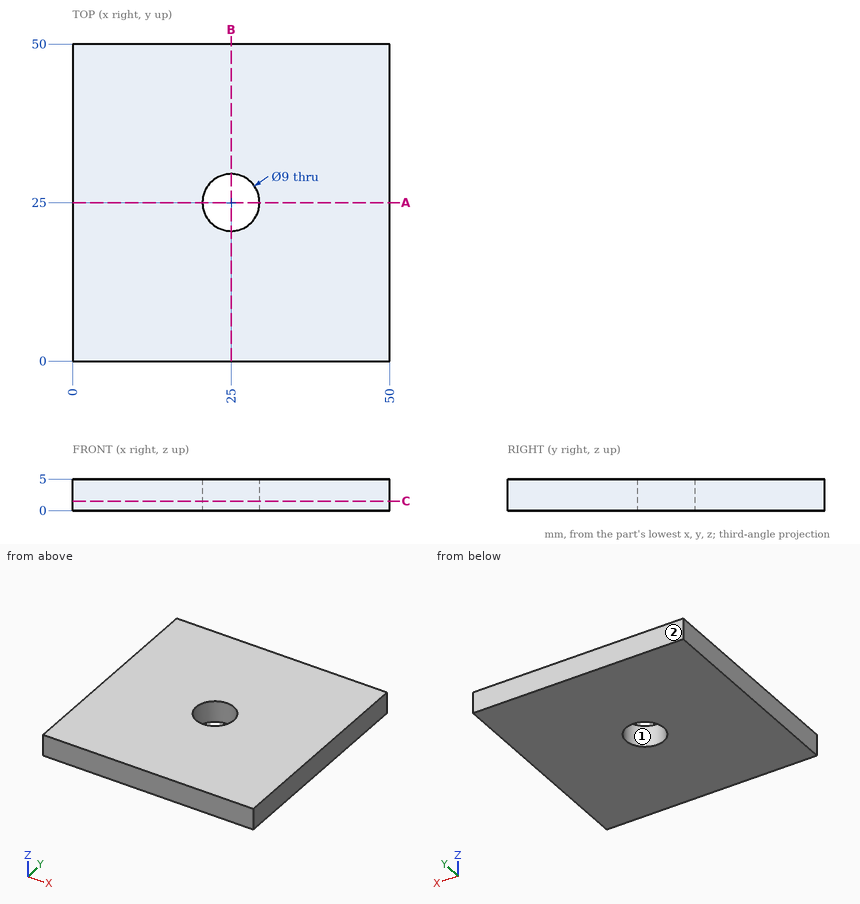
Drawing for the job (mm, zero at the part's lowest x, y, z). Give positions to 0.01 mm unless a question says otherwise; leave off trailing zeros. Loops run counter-clockwise (first coordinate to the right, second up) from the corner with the lowest first, then second, coordinate; pieces in that order, holes last. Notation, with made-up numbers: (-13, 76.5) - (18, 76.5) arc R14 cw to (18, 94.5) - close; hole circle Ø3 at (31, -25). An arc over 180 degrees is marked (long way). Write item = value, one per line. Start each with the question number.
1) Probe probe 1 along Y at (x, z) = (25, 3.35); probe 2 along Y at (x, z) = (28.5, 4.45); probe 3 along X at (y, z) = (23, 4.65). List the from-to ranges inside material, lowest first. Write a range as from..to.
2) Pull direction X, two halves, no side cores. Call the marked faces 1 and 2: +X half, -X half, draft (parallel to the pull), parting line (faces both ways), or undercut.
3) Band-saw the part on A-A on y = 25. Give the cut face in (x, z), plus the area to 3 significant figures.
4) Band-saw the part on C-C on z = 1.5. Give the cut face in (x, y).
5) Drop a flat-ended pin along its axis: pin 1 Ø14.5 at (x, y) = (25, 25) entering from +Z. Give the stop position or say it passes through.
Final values:
q1.probe_1 = 0..20.5, 29.5..50
q1.probe_2 = 0..22.17, 27.83..50
q1.probe_3 = 0..20.97, 29.03..50
q2.face_1 = undercut
q2.face_2 = draft
q3.outline = (0, 0) - (20.5, 0) - (20.5, 5) - (0, 5) - close; (29.5, 0) - (50, 0) - (50, 5) - (29.5, 5) - close
q3.area = 205 mm²
q4.outline = (0, 0) - (50, 0) - (50, 50) - (0, 50) - close; hole circle Ø9 at (25, 25)
q5.pin_1 = 5
